from build123d import *

# Parameters (mm, degrees)
EXTRUDE_1_DEPTH      = 7
EXTRUDE_1_DEPTH_BACK = 7


with BuildPart() as part:
    # 草圖1 → 填料-伸長1 (new, two sides: drawn at the far end of the back side and taken through both)
    with BuildSketch(Plane(origin=(0, 0, 0), x_dir=(0, 0, -1), z_dir=(1, 0, 0)).offset(-EXTRUDE_1_DEPTH_BACK)):
        with BuildLine():
            Line((-2.55, -4), (-2.55, -20.5))
            Line((-2.55, -20.5), (-2.25, -20.5))
            Line((-2.25, -20.5), (-2.25, -4))
            ThreePointArc((-2.25, -4), (-1.7, -3.45), (-1.15, -4))
            Line((-1.15, -4), (-0.85, -4))
            ThreePointArc((-0.85, -4), (-1.7, -3.15), (-2.55, -4))
        make_face()
    extrude(amount=EXTRUDE_1_DEPTH + EXTRUDE_1_DEPTH_BACK)


solid = part.part
Here's how the part is built. I have some questions about the finished solid (model axes, mm). Coordinates: 2 decimals unless noted, no trailing zeros. Order: outer loops, then holes, each group sorted by start corner. A loop starts at its lowest first (then second) coordinate and runs counter-clockwise, first axis right, second up. Notation, with made-up numbers: (88, 55.25) - (126, 55.25) arc R8 ccw to (126, 62.25) - close; hole circle Ø6 at (18.25, 34.5). An arc over 180 degrees is marked (long way). Use CSV: the item, a comma, the result in double quotes. Start each with the question number.
1. Suppose I cut it at C-C on y = -8.75. List the corners of the cut face in (x, z) for me, then the cut area to 3 significant figures.
2. I'm going to push a flat-ended pin straight in: pin 1 (8 mm diameter, centred on x = -0.5, y = -17, fed in from -Z). Where does the tip first touch, or does it pass through?
3. Please list where these lines run through material, in increasing order: line 1 (Z direction, x = 0.5, y = -7.25); line 2 (Y direction, x = -3.75, z = 1.7); line 3 (Y direction, x = -1, z = 2.35). Write a range as from..to.
4. If we mould it in two halves opening along Z, with no side actions, what happens to faces 1 (the face through (0, -12, 2.25)), 2 (the face through (0, -12, 2.55)), 3 (the face through (-0.1, -3.15, 1.68)), 4 (the face through (-0.1, -3.45, 1.71))? For each: +Z half, -Z half, draft (parallel to the pull), parting line (faces both ways), or undercut.
5. Suppose I cut it at A-A on x = -3.75. List the corners of the cut face in (y, z) for me, then the cut area to 3 significant figures.
6. Suppose I cut it at B-B on z = 1.7. List the corners of the cut face in (x, y) for me, then the cut area to 3 significant figures.
Output:
1,outline,"(-7, 2.25) - (7, 2.25) - (7, 2.55) - (-7, 2.55) - close"
1,area,"4.20 mm2"
2,pin 1,"stops at z = 2.25"
3,line 1,"z = 2.25..2.55"
3,line 2,"y = -3.45..-3.15"
3,line 3,"y = -20.5..-3.45"
4,face 1,"-Z half"
4,face 2,"+Z half"
4,face 3,"parting line"
4,face 4,"undercut"
5,outline,"(-20.5, 2.25) - (-4, 2.25) arc R0.55 cw to (-4, 1.15) - (-4, 0.85) arc R0.85 ccw to (-4, 2.55) - (-20.5, 2.55) - close"
5,area,"5.61 mm2"
6,outline,"(-7, -3.45) - (7, -3.45) - (7, -3.15) - (-7, -3.15) - close"
6,area,"4.20 mm2"
